```python
from build123d import *

# Parameters (mm, degrees)
SKETCH1_W           = 700
SKETCH1_H           = 200
SKETCH1_W_2         = 60
SKETCH1_H_2         = 140
BOSS_EXTRUDE1_DEPTH = 15


with BuildPart() as part:
    # Sketch1 → Boss-Extrude1 (new body)
    with BuildSketch(Plane(origin=(0, 0, 0), x_dir=(0, 0, -1), z_dir=(1, 0, 0))):
        with Locations((0, 100)):
            Rectangle(SKETCH1_W, SKETCH1_H)
        with Locations((-280, 100)):
            Rectangle(SKETCH1_W_2, SKETCH1_H_2, mode=Mode.SUBTRACT)
        with Locations((-168, 100)):
            Rectangle(SKETCH1_W_2, SKETCH1_H_2, mode=Mode.SUBTRACT)
        with Locations((-56, 100)):
            Rectangle(SKETCH1_W_2, SKETCH1_H_2, mode=Mode.SUBTRACT)
        with Locations((56, 100)):
            Rectangle(SKETCH1_W_2, SKETCH1_H_2, mode=Mode.SUBTRACT)
        with Locations((168, 100)):
            Rectangle(SKETCH1_W_2, SKETCH1_H_2, mode=Mode.SUBTRACT)
        with Locations((280, 100)):
            Rectangle(SKETCH1_W_2, SKETCH1_H_2, mode=Mode.SUBTRACT)
    extrude(amount=BOSS_EXTRUDE1_DEPTH)


solid = part.part
```
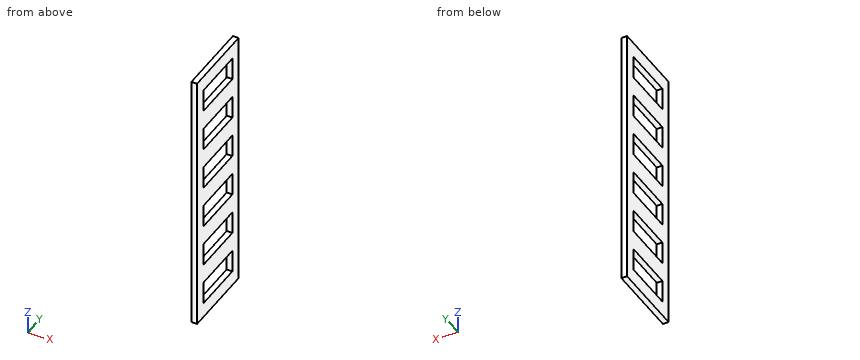
CAD build for the part. Positions are in the model's coordinates, mm. Round coordinates to 2 decimals unless told otherwise and drop trailing zeros. Write each loop counter-clockwise with the first axis right and the second up, starting at its lowest first coordinate (ties: lowest second). Pieces come first, ordered by that corner, then holes.
Item 1: Band-saw the part on B-B on y = 123. Write the cut outline in (x, z), then the cut area to 3 significant figures.
Filled in:
outline: (0, -350) - (15, -350) - (15, -310) - (0, -310) - close; (0, -250) - (15, -250) - (15, -198) - (0, -198) - close; (0, -138) - (15, -138) - (15, -86) - (0, -86) - close; (0, -26) - (15, -26) - (15, 26) - (0, 26) - close; (0, 86) - (15, 86) - (15, 138) - (0, 138) - close; (0, 198) - (15, 198) - (15, 250) - (0, 250) - close; (0, 310) - (15, 310) - (15, 350) - (0, 350) - close
area: 5,100 mm2
Item 2: Drill centre line: L1, parallel to Y at x = 12, z = 292.5. Where is it in solid material? Low to high.
Filled in:
L1: y = 0 to 30, 170 to 200
Item 3: Band-saw the part on C-C on x = 5.75. Write the cut outline in (y, z).
Filled in:
outline: (0, -350) - (200, -350) - (200, 350) - (0, 350) - close; hole (30, -310) - (170, -310) - (170, -250) - (30, -250) - close; hole (30, -198) - (170, -198) - (170, -138) - (30, -138) - close; hole (30, -86) - (170, -86) - (170, -26) - (30, -26) - close; hole (30, 26) - (170, 26) - (170, 86) - (30, 86) - close; hole (30, 138) - (170, 138) - (170, 198) - (30, 198) - close; hole (30, 250) - (170, 250) - (170, 310) - (30, 310) - close
Item 4: Band-saw the part on A-A on z = 264. Write the cut outline in (x, y), then the cut area to 3 significant figures.
Filled in:
outline: (0, 0) - (15, 0) - (15, 30) - (0, 30) - close; (0, 170) - (15, 170) - (15, 200) - (0, 200) - close
area: 900 mm2
